Here's how the part is built. I have some questions about the finished solid (model axes, mm). Face numbers are marked on the shaded views. A direction names the side the tool comes from. Round coordinates to 2 decimals unless told otherwise and drop trailing zeros. Write each loop counter-clockwise with the first axis right and the second up, starting at its lowest first coordinate (ties: lowest second). Pieces come first, ordered by that corner, then holes. Notation, with made-up numbers: (25.5, 13.25) -> (29.5, 13.25) arc R33 ccw to (29.5, 48.25) -> close; hole circle Ø8 at (-7, -25). An arc over 180 degrees is marked (long way). Answer as CSV lines item,"result".
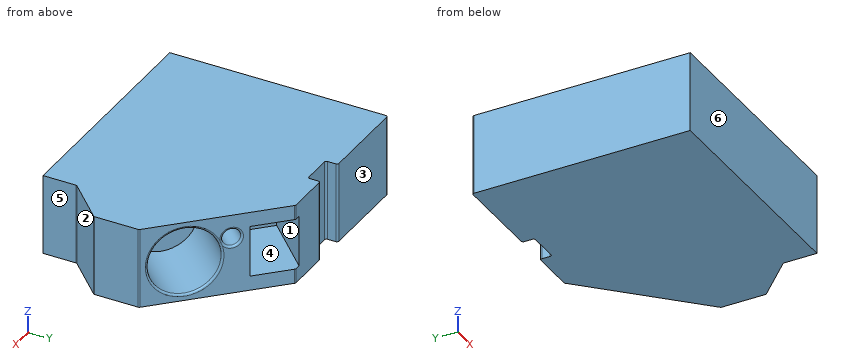
from build123d import *

# Parameters (mm, degrees)
EXTRUDE1_DEPTH = 9.9568
SKETCH2_R      = 4.191000000000001
SKETCH2_R_2    = 1.079499999999997
EXTRUDE2_DEPTH = 9.144
FILLET1_R      = 0.254


with BuildPart() as part:
    # Sketch1 → Extrude1 (new body)
    with BuildSketch(Plane.XY):
        with BuildLine():
            Line((0, 0), (0, 26.720799999999993))
            ThreePointArc((0, 26.720799999999993), (0.07439487757861757, 26.900405122421375), (0.2540000000000018, 26.974799999999995))
            Line((0.2540000000000018, 26.974799999999995), (11.048999999999998, 26.9748))
            ThreePointArc((11.048999999999998, 26.9748), (11.228605122421383, 26.900405122421382), (11.303, 26.720799999999997))
            Line((11.303, 26.720799999999997), (11.303, 25.704799999999995))
            ThreePointArc((11.303, 25.704799999999995), (11.377394877578618, 25.52519487757861), (11.557000000000002, 25.450799999999994))
            Line((11.557000000000002, 25.450799999999994), (15.036799999999998, 25.450799999999994))
            ThreePointArc((15.036799999999998, 25.450799999999994), (15.216405122421383, 25.52519487757861), (15.2908, 25.704799999999995))
            Line((15.2908, 25.704799999999995), (15.2908, 26.720799999999997))
            ThreePointArc((15.2908, 26.720799999999997), (15.365194877578617, 26.900405122421382), (15.5448, 26.9748))
            Line((15.5448, 26.9748), (20.72278975515723, 26.974800000000002))
            ThreePointArc((20.72278975515723, 26.974800000000002), (20.819991346977968, 26.955465401257868), (20.902394877578615, 26.90040512242138))
            Line((20.902394877578615, 26.90040512242138), (33.275805122421374, 14.52699487757856))
            ThreePointArc((33.275805122421374, 14.52699487757856), (33.33086540125785, 14.444591346977912), (33.350199999999994, 14.347389755157183))
            Line((33.350199999999994, 14.347389755157183), (33.35019999999999, 8.969810244842721))
            ThreePointArc((33.35019999999999, 8.969810244842721), (33.33086540125785, 8.872608653021988), (33.275805122421374, 8.790205122421336))
            Line((33.275805122421374, 8.790205122421336), (28.72762045926646, 4.242020459266578))
            ThreePointArc((28.72762045926646, 4.242020459266578), (28.67256018042997, 4.159616928665926), (28.653225581687842, 4.0624153368451905))
            Line((28.653225581687842, 4.0624153368451905), (28.653225581687938, 4.34e-15))
            Line((28.653225581687938, 4.34e-15), (0, 0))
        make_face()
    extrude(amount=EXTRUDE1_DEPTH)

    # Sketch2 → Extrude2 (cut)
    with BuildSketch(Plane(origin=(23.90140000000005, 23.90139999999994, 0), x_dir=(0, 0, -1), z_dir=(0.7071067811865491, 0.707106781186546, 0))):
        with Locations(Location((-4.978399999999999, -8.204766282245217, 0), (0, 0, 90))):
            Circle(SKETCH2_R)
        with Locations(Location((-7.073900000000001, -2.887802416466178, 0), (0, 0, 90))):
            Circle(SKETCH2_R_2)
        Polygon((-8.153400000000001, 4.876233717754782), (-1.8034000000000028, 4.876233717754782), (-1.803400000000002, -0.838766282245218), (-8.153400000000001, -0.838766282245218), align=None)
    extrude(amount=-EXTRUDE2_DEPTH, mode=Mode.SUBTRACT)

    # Fillet1
    # the kernel refuses this fillet: 0.254 mm, written as the material it takes off along each edge
    with BuildSketch(Plane(origin=(29.70304587622637, 18.099754123773593, 4.978399999999999), x_dir=(-0.7071067811865458, 0.7071067811865491, 0), z_dir=(0, 0, -1))) as fillet1_piece_1:
        with BuildLine():
            CenterArc((4.191000000000001 + FILLET1_R, -FILLET1_R), FILLET1_R, 89.99999999999982, 89.9999999999984)
            Line((4.190999999999995, -FILLET1_R), (4.191000000000001, 1e-16))
            Line((4.191000000000001, 1e-16), (4.191000000000001 + FILLET1_R, -8.03e-15))
        make_face()
    revolve(axis=Axis((29.70304587622637, 18.099754123773593, 4.978399999999999), (0.7071067811865491, 0.707106781186546, 0)), mode=Mode.SUBTRACT)
    with BuildSketch(Plane(origin=(25.94338467141018, 21.8594153285898, 7.073900000000001), x_dir=(-0.7071067811865476, 0.7071067811865476, 0), z_dir=(0, 0, -1.0000000000000002))) as fillet1_piece_2:
        with BuildLine():
            CenterArc((1.079499999999997 + FILLET1_R, -FILLET1_R), FILLET1_R, 90, 89.99999999999832)
            Line((1.0794999999999895, -FILLET1_R), (1.079499999999997, -3e-17))
            Line((1.079499999999997, -3e-17), (1.079499999999997 + FILLET1_R, -5.05e-15))
        make_face()
    revolve(axis=Axis((25.94338467141018, 21.8594153285898, 7.073900000000001), (0.7071067811865491, 0.707106781186546, 0)), mode=Mode.SUBTRACT)


solid = part.part
Item 1: Suppose I cut it at B-B, the plane y = 2. List the corners of the cut face in (x, z) for me.
Results found:
outline,"(0, 0) -> (28.65, 0) -> (28.65, 9.96) -> (0, 9.96) -> close"
Item 2: Suppose I cut it at C-C, the plane x = 12. List the corners of the cut face in (y, z) for me, then the cut area to 3 significant figures.
Results found:
outline,"(0, 0) -> (25.45, 0) -> (25.45, 9.96) -> (0, 9.96) -> close"
area,"253 mm²"
Item 3: Suppose I cut it at D-D, the plane x = 23. State how many separate pieces and enclosed holes the cut face has, then the cut area to 3 significant figures.
Results found:
separate pieces,"1"
enclosed holes,"2"
area,"188 mm²"
Item 4: If we mould it in two halves opening along Y, with no side actions, what happens to the marked faces 3, 4, 5 and 6? For each: pulls with the +Y half, pulls with the -Y half, needs draft (parallel to the pull), parting line crosses it, or undercut.
Results found:
face 3,"pulls with the +Y half"
face 4,"undercut"
face 5,"needs draft"
face 6,"pulls with the -Y half"
Item 5: For the marked faces 1 and 2, which set-ups out of +Z, -Z, +X, -X, +Y, -Y let a thin tool reach every point of the face, with its end or its side?
Results found:
face 1,"none"
face 2,"+Z, -Z, +X, -Y"
Item 6: Will these pins go through, and if not, where does the flat tip stop? pin 1 (2 mm diameter, centred on y = 20, z = 5.5, fed in from +X); pin 2 (3 mm diameter, centred on x = 14, z = 7.5, fed in from +Y); pin 3 (1.5 mm diameter, centred on y = 22, z = 2, fed in from +X).
Results found:
pin 1,"stops at x = 26.7"
pin 2,"stops at y = 26.97"
pin 3,"stops at x = 26.55"
Item 7: I need wall thicknesses on L1, parallel to Z at x = 24, y = 23.25; L2, parallel to X at y = 17.5, z = 6.5; L3, parallel to X at y = 4.25, z = 0.75. Which ranges of each line are inside material? Lowest first, please.
Results found:
L1,"z = 0 to 1.8, 8.15 to 9.96"
L2,"x = 0 to 17.37, 18.69 to 20.29, 22.88 to 23.58"
L3,"x = 0 to 28.74"
Item 8: Suppose I cut it at A-A, the plane x = 17.5. List the corners of the cut face in (y, z) for me.
Results found:
outline,"(0, 0) -> (26.97, 0) -> (26.97, 9.96) -> (0, 9.96) -> close; hole (17.37, 1.8) -> (24.4, 1.8) -> (24.4, 8.15) -> (17.37, 8.15) -> close"
